Can you work these out from the model? Positions are in its coordinate system, mm. Face numbers are marked on the shaded views. A direction names the side the tool comes from. Give positions to 0.01 mm unless a question says otherwise; leave off trailing zeros. Loops run counter-clockwise (first coordinate to the right, second up) from the corner with the lowest first, then second, coordinate; pieces in that order, holes last. Notation, with made-up numbers: (42, 10) - (55, 10) arc R14 ccw to (55, 37) - close; hole circle Ø8 at (20.5, 74). An arc over 180 degrees is marked (long way). Answer as a JSON object with one key per item and string values. Group by question number.
Item 1: Suppose I cut it at C-C on y = 0. Write out the boundary of the cut face in (x, z), and give its area (3 significant figures).
Item 2: Suppose I cut it at A-A on x = 0. Write out the boundary of the cut face in (y, z).
Item 3: Suppose I cut it at B-B on z = 5. Write out the boundary of the cut face in (x, y).
Item 4: Suppose I cut it at D-D on z = -7.5. Write out the boundary of the cut face in (x, y), and give its area (3 significant figures).
Item 5: Which directions (+Z, -Z, +X, -X, +Y, -Y) give clear straight access to the entire face, cutting with the end or side of a thin tool? Please do the marked faces 1, 2, 3 and 4.
Item 6: Thinking about a two-plate mould opening in Z: for the marked faces 5, 6, 7 and 8, which applies, pulls with the +Z half, pulls with the -Z half, needs draft (parallel to the pull), parting line crosses it, or undercut?
Item 7: Please list where these lines run through material, in increasing order: L1, parallel to Y at x = -12.5, z = 1.5; L2, parallel to Y at x = 0, z = 4.75; L3, parallel to Z at x = 0, y = 2.7.
Item 8: Will these pins go through, and if not, where does the flat tip stop? pin 1 (5 mm diameter, centred on y = 4.5, z = -11.5, fed in from -X); pin 2 (1 mm diameter, centred on x = 6, z = -11, fed in from -Y); pin 3 (2.5 mm diameter, centred on x = 0, z = -10, fed in from +Y); pin 4 (2.5 mm diameter, centred on x = -11.48, z = 5, fed in from -Y).
from build123d import *

# Parameters (mm, degrees)
F1_DEPTH  = 10
F2_R      = 7.5
F3_DEPTH  = 15
F4_R      = 2.5
F5_DEPTH  = 10
F6_R      = 1.5
F7_DEPTH  = 25
F8_R      = 1.514445
F9_DEPTH  = 25
F10_W     = 6.295164
F10_H     = 2.4
F11_DEPTH = 8


with BuildPart() as f1:
    # F0 (on Top) → F1 (new body)
    with BuildSketch(Plane.XY):
        with BuildLine():
            Line((-14.676502, -3.500946), (-8.291163, -3.500946))
            ThreePointArc((-8.291163, -3.500946), (9, 0), (-8.291163, 3.500946))
            Line((-8.291163, 3.500946), (-14.676502, 3.500946))
            Line((-14.676502, 3.500946), (-14.676502, 0.713968))
            Line((-14.676502, 0.713968), (-3.935766, 0.713968))
            ThreePointArc((-3.935766, 0.713968), (4, 0), (-3.935766, -0.713968))
            Line((-3.935766, -0.713968), (-14.676502, -0.713968))
            Line((-14.676502, -0.713968), (-14.676502, -3.500946))
        make_face()
    extrude(amount=F1_DEPTH)

    # F2 (on face) → F3 (join)
    with BuildSketch(Plane(origin=(0, 0, 0), x_dir=(1, 0, 0), z_dir=(0, 0, -1))):
        Circle(F2_R)
    extrude(amount=F3_DEPTH)

    # F4 (on face) → F5 (cut)
    with BuildSketch(Plane(origin=(0, 0, -15), x_dir=(1, 0, 0), z_dir=(0, 0, -1))):
        Circle(F4_R)
    extrude(amount=-F5_DEPTH, mode=Mode.SUBTRACT)

    # F6 (on face) → F7 (cut)
    with BuildSketch(Plane.XZ.offset(3.500946)):
        with Locations((-11.483832, 5)):
            Circle(F6_R)
    extrude(amount=-F7_DEPTH, mode=Mode.SUBTRACT)

    # F8 (on Front) → F9 (cut)
    with BuildSketch(Plane.XZ):
        with Locations((0, -10.001184)):
            Circle(F8_R)
    extrude(amount=-F9_DEPTH, mode=Mode.SUBTRACT)

    # F10 (on face) → F11 (cut)
    with BuildSketch(Plane(origin=(0, 0, -15), x_dir=(1, 0, 0), z_dir=(0, 0, -1))):
        with Locations((0, -4.299535)):
            Rectangle(F10_W, F10_H)
    extrude(amount=-F11_DEPTH, mode=Mode.SUBTRACT)


solid = f1.part
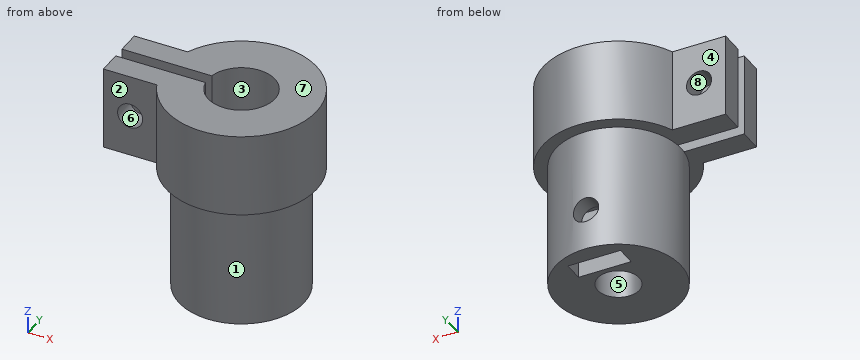
Worked out:
{
 "1": {"outline": "(-7.5, -15) - (-2.5, -15) - (-2.5, -5) - (2.5, -5) - (2.5, -15) - (7.5, -15) - (7.5, 0) - (9, 0) - (9, 10) - (4, 10) - (4, 0) - (-7.5, 0) - close", "area": "225 mm2"},
 "2": {"outline": "(-9, 0) - (-7.5, 0) - (-7.5, -15) - (-2.5, -15) - (-2.5, -5) - (2.5, -5) - (2.5, -8.49) - (3.1, -8.49) - (3.1, -7) - (5.5, -7) - (5.5, -8.49) - (7.5, -8.49) - (7.5, 0) - (9, 0) - (9, 10) - (4, 10) - (4, 0) - (-4, 0) - (-4, 10) - (-9, 10) - close; (2.5, -15) - (3.1, -15) - (3.1, -11.52) - (2.5, -11.52) - close; (5.5, -15) - (7.5, -15) - (7.5, -11.52) - (5.5, -11.52) - close"},
 "3": {"outline": "(-14.68, -3.5) - (-12.98, -3.5) - (-12.98, -0.71) - (-14.68, -0.71) - close; (-14.68, 0.71) - (-12.98, 0.71) - (-12.98, 3.5) - (-14.68, 3.5) - close; (-9.98, -3.5) - (-8.29, -3.5) arc R9 ccw (long way) to (-8.29, 3.5) - (-9.98, 3.5) - (-9.98, 0.71) - (-3.94, 0.71) arc R4 cw (long way) to (-3.94, -0.71) - (-9.98, -0.71) - close"},
 "4": {"outline": "circle Ø15 at (0, 0); hole (-3.15, 3.1) - (3.15, 3.1) - (3.15, 5.5) - (-3.15, 5.5) - close; hole circle Ø5 at (0, 0)", "area": "142 mm2"},
 "5": {"face 1": "-Z", "face 2": "+Z, -Z, -X, -Y", "face 3": "+Z", "face 4": "+Z, -Z, -X, +Y"},
 "6": {"face 5": "needs draft", "face 6": "undercut", "face 7": "pulls with the +Z half", "face 8": "undercut"},
 "7": {"L1": "y = -3.5 to -0.71, 0.71 to 3.5", "L2": "y = -9 to -4, 4 to 9", "L3": "z = -15 to -11.52, -8.49 to 0"},
 "8": {"pin 1": "stops at x = -7.23", "pin 2": "stops at y = -5.1", "pin 3": "stops at y = -2.17", "pin 4": "passes through"}
}
